Autodesk Inventor part; units mm, degrees
ref_plane "YZ Plane" through (0, 0, 0) normal (1, 0, 0) x (0, 1, 0)
ref_plane "XZ Plane" through (0, 0, 0) normal (0, 1, 0) x (-1, 0, 0)
ref_plane "XY Plane" through (0, 0, 0) normal (0, 0, 1) x (1, 0, 0)
sketch "Sketch1" plane through (0, 0, 0) normal (0, 1, 0) x (-1, 0, 0)
  line L0 (20, 20) -> (20, -20)
  line L1 (20, -20) -> (-20, -20)
  line L2 (-20, -20) -> (-20, 20)
  line L3 (-20, 20) -> (20, 20)
  line L4 (-15, 15) -> (-15, -15) construction
  line L5 (-15, -15) -> (15, -15) construction
  line L6 (15, -15) -> (15, 15) construction
  line L7 (15, 15) -> (-15, 15) construction
  circle A0 centre (15, 15) radius 3.05
  circle A1 centre (15, -15) radius 3.05
  circle A2 centre (-15, -15) radius 3.05
  circle A3 centre (-15, 15) radius 3.05
  line L8 (0, 0) -> (-18.5703, 0) construction
  line L9 (-8, 2.3333) -> (-8, 9)
  line L10 (-10, 11) -> (-12, 11)
  line L11 (-14, 9) -> (-14, -9)
  line L12 (-12, -11) -> (-10, -11)
  line L13 (-8, -9) -> (-8, -2.3333)
  line L14 (8, -2.3333) -> (8, -9)
  line L15 (10, -11) -> (12, -11)
  line L16 (14, -9) -> (14, 9)
  line L17 (12, 11) -> (10, 11)
  line L18 (8, 9) -> (8, 2.3333)
  line L19 (0, 0) -> (0, 18.05) construction
  line L20 (0, 0) -> (-18.05, 0) construction
  arc A4 (-12, 11) -> (-14, 9) centre (-12, 9) ccw
  arc A5 (-8, 9) -> (-10, 11) centre (-10, 9) ccw
  arc A6 (-10, -11) -> (-8, -9) centre (-10, -9) ccw
  arc A7 (-14, -9) -> (-12, -11) centre (-12, -9) ccw
  arc A8 (8, -9) -> (10, -11) centre (10, -9) ccw
  arc A9 (12, -11) -> (14, -9) centre (12, -9) ccw
  arc A10 (14, 9) -> (12, 11) centre (12, 9) ccw
  arc A11 (10, 11) -> (8, 9) centre (10, 9) ccw
  line L21 (8, 2.3333) -> (4, 2.3333)
  line L22 (4, 2.3333) -> (4, 4.3333)
  line L23 (2, 6.3333) -> (-2, 6.3333)
  line L24 (-4, 4.3333) -> (-4, 2.3333)
  line L25 (-4, 2.3333) -> (-8, 2.3333)
  line L26 (-8, -2.3333) -> (-4, -2.3333)
  line L27 (-4, -2.3333) -> (-4, -4.3333)
  line L28 (-2, -6.3333) -> (2, -6.3333)
  line L29 (4, -4.3333) -> (4, -2.3333)
  line L30 (4, -2.3333) -> (8, -2.3333)
  arc A12 (4, 4.3333) -> (2, 6.3333) centre (2, 4.3333) ccw
  arc A13 (-2, 6.3333) -> (-4, 4.3333) centre (-2, 4.3333) ccw
  arc A14 (-4, -4.3333) -> (-2, -6.3333) centre (-2, -4.3333) ccw
  arc A15 (2, -6.3333) -> (4, -4.3333) centre (2, -4.3333) ccw
  point P0 (-8, 11)
  point P1 (-14, 11)
  point P2 (-8, -11)
  point P3 (8, -11)
  point P4 (14, -11)
  point P5 (8, 11)
  point P6 (4, 6.3333)
  point P7 (-4, 6.3333)
  point P8 (-4, -6.3333)
  point P9 (4, -6.3333)
  dimension "d0" = 40
  dimension "d1" = 40
  dimension "d2" = 30
  dimension "d3" = 6.1
  dimension "d53" = 20
  dimension "d54" = 15
  dimension "d57" = 8
  dimension "d58" = 16
  dimension "d59" = 22
  dimension "d60" = 6
  dimension "d61" = 2
  dimension "d96" = 4.6667
  dimension "d97" = 2.3333
  dimension "d98" = 4
  dimension "d99" = 8
  dimension "d100" = 8
  dimension "d101" = 4
  dimension "d102" = 2
extrude "Extrusion5" add sketch "Sketch1" along normal blind 8
sketch "Sketch8" plane through (-20, 0, 20) normal (0, 0, 1) x (1, 0, 0)
  circle A0 centre (20, 4) radius 1.5
  line L0 (40, 0) -> (0, 0)
  point P0 (20, 0)
  dimension "d103" = 3
  dimension "d104" = 4
sketch "Sketch9" plane through (20, 0, 20) normal (1, 0, 0) x (0, 0, -1)
  line L0 (40, 0) -> (0, 0)
  line L1 (40, 0) -> (40, 8)
  line L2 (0, 8) -> (40, 8)
  line L3 (0, 0) -> (0, 8)
  point P0 (20, 0)
  point P1 (5, 4)
  point P2 (35, 4)
  dimension "d107" = 5
  dimension "d108" = 5
  dimension "d109" = 4
  dimension "d110" = 4
hole "Hole1" at (20, 4, 15) at (20, 4, -15) direction (-1, 0, 0) diameter 2.013 depth 5 tip angle 118
sketch "Sketch10" plane through (-20, 0, -20) normal (-1, 0, 0) x (0, 0, 1)
  circle A0 centre (35, 4) radius 1.0065
  circle A1 centre (5, 4) radius 1.0065
  point P0 (20, 0)
  point P1 (33.9935, 4)
  point P2 (3.9935, 4)
hole "Hole2" at (-20, 4, 15) at (-20, 4, -15) direction (1, 0, 0) diameter 2.013 depth 5 tip angle 118
hole "Hole3" at (0, 4, 20) direction (0, 0, -1) diameter 3.1 end through all
equation "\"d1\" = d0"
properties part number "HolderThin2"
Source: CAD feature listing. Evaluate the final solid. Frame: model axes, mm. A direction names the side the tool comes from. Give positions to 0.01 mm unless a question says otherwise; leave off trailing zeros. Order: outer loops, then holes, each group sorted by start corner. A loop starts at its lowest first (then second) coordinate and runs counter-clockwise, first axis right, second up.
(1) Section query C-C (x = 6.5). Return the cut outline in (y, z), plus the area to 3 significant figures.
(2) Access query for faces 1 (the face through (-18.925, 3.956, 13.994)), 2 (the face through (3.4, 3.94, -5.76)), 3 (the face through (18.925, 3.956, -13.994)). Directions: +Z, -Z, +X, -X, +Y, -Y. A direction counts if a zero-diameter tool reaches every point of the face in a straight line with its end or side. Return the directions, or none.
(3) Section query B-B (x = 0). Return the cut outline in (y, z).
(4) Material intervals for line 1 along Z through (x, y) = (-15, 1.5); line 2 along X through (y, z) = (2.75, 3.5); line 3 along X through (y, z) = (6.5, -0.5), sorted ascending.
(5) Contact query for flat-ended pins moving along their axis: P1, Ø4, axis at x = 0, z = 11, coming from the -Y side; P2, Ø2.5, axis at x = 0, y = 4, coming from the +Z side. Output: stop coordinate, or through.
(6) Section query D-D (z = 0). Return the cut outline in (x, y).
(7) Pull-direction query (Z, two-part tool) for faces 4 (the face through (-8, 4, -6)), 5 (the face through (8.57, 3.94, -10.4)), 6 (the face through (0, 2, -20)), 7 (the face through (5, 8, 5)); classes: +Z half, -Z half, draft (parallel to the pull), parting line (faces both ways), or undercut.
(8) Section query A-A (z = 15). Return the cut outline in (x, y).
Outcome:
1. outline: (0, -20) - (8, -20) - (8, -2.33) - (0, -2.33) - close; (0, 2.33) - (8, 2.33) - (8, 20) - (0, 20) - close
1. area: 283 mm2
2. face 1: -X
2. face 2: +Y, -Y
2. face 3: +X
3. outline: (0, -20) - (2.45, -20) - (2.45, -6.33) - (0, -6.33) - close; (0, 6.33) - (2.45, 6.33) - (2.45, 20) - (0, 20) - close; (5.55, -20) - (8, -20) - (8, -6.33) - (5.55, -6.33) - close; (5.55, 6.33) - (8, 6.33) - (8, 20) - (5.55, 20) - close
4. line 1: z = -20 to -18.05, -11.95 to 11.95, 18.05 to 20
4. line 2: x = -20 to -14, -8 to -4, 4 to 8, 14 to 20
4. line 3: x = -20 to -14, 14 to 20
5. P1: stops at y = 0
5. P2: passes through
6. outline: (-20, 0) - (-14, 0) - (-14, 8) - (-20, 8) - close; (14, 0) - (20, 0) - (20, 8) - (14, 8) - close
7. face 4: undercut
7. face 5: undercut
7. face 6: -Z half
7. face 7: draft
8. outline: (-20, 0) - (-18.05, 0) - (-18.05, 2.99) - (-20, 2.99) - close; (-20, 5.01) - (-18.05, 5.01) - (-18.05, 8) - (-20, 8) - close; (-11.95, 0) - (11.95, 0) - (11.95, 8) - (-11.95, 8) - close; (18.05, 0) - (20, 0) - (20, 2.99) - (18.05, 2.99) - close; (18.05, 5.01) - (20, 5.01) - (20, 8) - (18.05, 8) - close; hole circle Ø3.1 at (0, 4)
